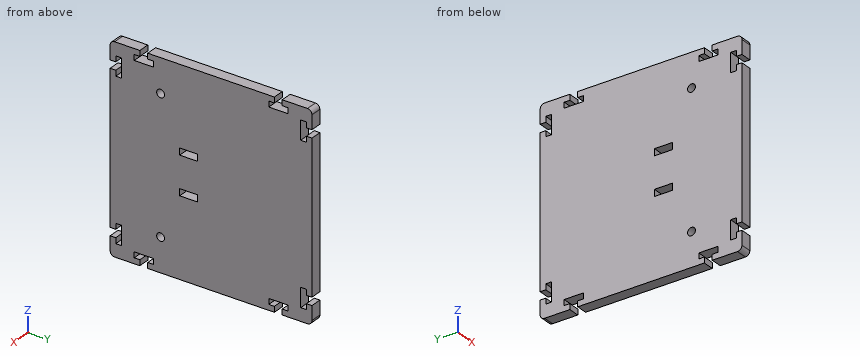
```python
from build123d import *

# Parameters (mm, degrees)
SKETCH_1_R      = 1.75
SKETCH_1_W      = 3
SKETCH_1_H      = 8
EXTRUDE_1_DEPTH = 5


with BuildPart() as part:
    # Эскиз1 → Бобышка-Вытянуть1 (new body)
    with BuildSketch(Plane(origin=(0, 0, 0), x_dir=(0, 0, -1), z_dir=(1, 0, 0))):
        with BuildLine():
            Line((-36.75, 45), (-36.75, 42.5))
            Line((-36.75, 42.5), (-39.25, 42.5))
            Line((-39.25, 42.5), (-39.25, 40))
            Line((-39.25, 40), (-30.75, 40))
            Line((-30.75, 40), (-30.75, 42.5))
            Line((-30.75, 42.5), (-33.25, 42.5))
            Line((-33.25, 42.5), (-33.25, 45))
            Line((-33.25, 45), (33.25, 45))
            Line((33.25, 45), (33.25, 42.5))
            Line((33.25, 42.5), (30.75, 42.5))
            Line((30.75, 42.5), (30.75, 40))
            Line((30.75, 40), (39.25, 40))
            Line((39.25, 40), (39.25, 42.5))
            Line((39.25, 42.5), (36.75, 42.5))
            Line((36.75, 42.5), (36.75, 45))
            Line((36.75, 45), (43, 45))
            ThreePointArc((43, 45), (44.414213562, 44.414213562), (45, 43))
            Line((45, 43), (45, 31.75))
            Line((45, 31.75), (42.5, 31.75))
            Line((42.5, 31.75), (42.5, 34.25))
            Line((42.5, 34.25), (40, 34.25))
            Line((40, 34.25), (40, 25.75))
            Line((40, 25.75), (42.5, 25.75))
            Line((42.5, 25.75), (42.5, 28.25))
            Line((42.5, 28.25), (45, 28.25))
            Line((45, 28.25), (45, -28.25))
            Line((45, -28.25), (42.5, -28.25))
            Line((42.5, -28.25), (42.5, -25.75))
            Line((42.5, -25.75), (40, -25.75))
            Line((40, -25.75), (40, -34.25))
            Line((40, -34.25), (42.5, -34.25))
            Line((42.5, -34.25), (42.5, -31.75))
            Line((42.5, -31.75), (45, -31.75))
            Line((45, -31.75), (45, -43))
            ThreePointArc((45, -43), (44.414213562, -44.414213562), (43, -45))
            Line((43, -45), (36.75, -45))
            Line((36.75, -45), (36.75, -42.5))
            Line((36.75, -42.5), (39.25, -42.5))
            Line((39.25, -42.5), (39.25, -40))
            Line((39.25, -40), (30.75, -40))
            Line((30.75, -40), (30.75, -42.5))
            Line((30.75, -42.5), (33.25, -42.5))
            Line((33.25, -42.5), (33.25, -45))
            Line((33.25, -45), (-33.25, -45))
            Line((-33.25, -45), (-33.25, -42.5))
            Line((-33.25, -42.5), (-30.75, -42.5))
            Line((-30.75, -42.5), (-30.75, -40))
            Line((-30.75, -40), (-39.25, -40))
            Line((-39.25, -40), (-39.25, -42.5))
            Line((-39.25, -42.5), (-36.75, -42.5))
            Line((-36.75, -42.5), (-36.75, -45))
            Line((-36.75, -45), (-43, -45))
            ThreePointArc((-43, -45), (-44.414213562, -44.414213562), (-45, -43))
            Line((-45, -43), (-45, -31.75))
            Line((-45, -31.75), (-42.5, -31.75))
            Line((-42.5, -31.75), (-42.5, -34.25))
            Line((-42.5, -34.25), (-40, -34.25))
            Line((-40, -34.25), (-40, -25.75))
            Line((-40, -25.75), (-42.5, -25.75))
            Line((-42.5, -25.75), (-42.5, -28.25))
            Line((-42.5, -28.25), (-45, -28.25))
            Line((-45, -28.25), (-45, 28.25))
            Line((-45, 28.25), (-42.5, 28.25))
            Line((-42.5, 28.25), (-42.5, 25.75))
            Line((-42.5, 25.75), (-40, 25.75))
            Line((-40, 25.75), (-40, 34.25))
            Line((-40, 34.25), (-42.5, 34.25))
            Line((-42.5, 34.25), (-42.5, 31.75))
            Line((-42.5, 31.75), (-45, 31.75))
            Line((-45, 31.75), (-45, 43))
            ThreePointArc((-45, 43), (-44.414213562, 44.414213562), (-43, 45))
            Line((-43, 45), (-36.75, 45))
        make_face()
        with Locations((-30, -22.5)):
            Circle(SKETCH_1_R, mode=Mode.SUBTRACT)
        with Locations((30, -22.5)):
            Circle(SKETCH_1_R, mode=Mode.SUBTRACT)
        with Locations((8.5, -10)):
            Rectangle(SKETCH_1_W, SKETCH_1_H, mode=Mode.SUBTRACT)
        with Locations((-8.5, -10)):
            Rectangle(SKETCH_1_W, SKETCH_1_H, mode=Mode.SUBTRACT)
    extrude(amount=EXTRUDE_1_DEPTH)


solid = part.part
```
Model file for the job. Use its own axes, mm. Round coordinates to 2 decimals unless told otherwise and drop trailing zeros. Loops run counter-clockwise (first coordinate to the right, second up) from the corner with the lowest first, then second, coordinate; pieces in that order, holes last. Notation, with made-up numbers: M -25.75,35.5 L -9.75,35.5 A14 cw -9.75,54.5 Z; hole C 80,35 d2. An arc over 180 degrees is marked long. Put each result on its own line as item: value. Start each with the question number.
Item 1: Cut at A-A (z = 8.5). List the corners of the cut face in (x, y).
Item 2: Drop flat-ended pins along their axis: P1, Ø1.2, axis at x = 2, z = 44, coming from the +Y side; P2, Ø1.2, axis at x = 1.5, y = -44.5, coming from the +Z side. Give the stop position or say it passes through.
Item 3: Cut at C-C (x = 2.1). Give the number of separate pieces and of enclosed holes in the cut face, then the cut area to 3 significant figures.
Item 4: Cut at B-B (y = -22.5). List the corners of the cut face in (x, z).
Item 5: Drill centre lines: line 1 along Z through (x, y) = (0.45, 26.5); line 2 along Y through (x, z) = (1.45, 30); line 3 along Z through (x, y) = (2.75, -21). Where is each one in solid material? Low to high.
Answer block:
1. outline: M 0,-45 L 5,-45 L 5,-14 L 0,-14 Z; M 0,-6 L 5,-6 L 5,45 L 0,45 Z
2. P1: y = 44.96
2. P2: z = 44.79
3. separate pieces: 1
3. enclosed holes: 4
3. area: 7,790 mm2
4. outline: M 0,-45 L 5,-45 L 5,-31.75 L 0,-31.75 Z; M 0,-28.25 L 5,-28.25 L 5,28.25 L 0,28.25 Z; M 0,31.75 L 5,31.75 L 5,45 L 0,45 Z
5. line 1: -45 to -42.5, -40 to 40, 42.5 to 45
5. line 2: -45 to -24.25, -20.75 to 45
5. line 3: -45 to -30.9, -29.1 to 29.1, 30.9 to 45
